```python
from build123d import *

# Parameters (mm, degrees)
F0_W     = 80
F0_H     = 55
F1_DEPTH = 10
F2_W     = 10
F2_H     = 10
F3_DEPTH = 5
F4_R     = 1


with BuildPart() as f1:
    # F0 (on Front) → F1 (new body)
    with BuildSketch(Plane.XZ):
        with Locations((-69.614079, 6.646032)):
            Rectangle(F0_W, F0_H)
    extrude(amount=F1_DEPTH)

    # F2 (on face) → F3 (cut)
    with BuildSketch(Plane.XZ.offset(10)):
        with Locations((-94.614079, 19.146032)):
            Rectangle(F2_W, F2_H)
        with Locations((-94.614079, -4.553968)):
            Rectangle(F2_W, F2_H)
        with Locations((-69.614079, 19.146032)):
            Rectangle(F2_W, F2_H)
        with Locations((-69.614079, -4.553968)):
            Rectangle(F2_W, F2_H)
        with Locations((-44.614079, 19.146032)):
            Rectangle(F2_W, F2_H)
        with Locations((-44.614079, -4.553968)):
            Rectangle(F2_W, F2_H)
    extrude(amount=-F3_DEPTH, mode=Mode.SUBTRACT)

    # F4
    f4_edges = [f1.edges().sort_by_distance(p)[0] for p in [
        (-69.614079, -10, 34.146032),
        (-29.614079, -10, 6.646032),
        (-109.614079, -10, 6.646032),
        (-69.614079, -10, -20.853968),
        (-89.614079, -10, -4.553968),
        (-94.614079, -10, 0.446032),
        (-99.614079, -10, -4.553968),
        (-94.614079, -10, -9.553968),
        (-64.614079, -10, -4.553968),
        (-69.614079, -10, 0.446032),
        (-74.614079, -10, -4.553968),
        (-69.614079, -10, -9.553968),
        (-39.614079, -10, -4.553968),
        (-44.614079, -10, 0.446032),
        (-49.614079, -10, -4.553968),
        (-44.614079, -10, -9.553968),
        (-89.614079, -10, 19.146032),
        (-94.614079, -10, 24.146032),
        (-99.614079, -10, 19.146032),
        (-94.614079, -10, 14.146032),
        (-64.614079, -10, 19.146032),
        (-69.614079, -10, 24.146032),
        (-74.614079, -10, 19.146032),
        (-69.614079, -10, 14.146032),
        (-39.614079, -10, 19.146032),
        (-44.614079, -10, 24.146032),
        (-49.614079, -10, 19.146032),
        (-44.614079, -10, 14.146032),
        (-69.614079, 0, 34.146032),
        (-109.614079, 0, 6.646032),
        (-69.614079, 0, -20.853968),
        (-29.614079, 0, 6.646032),
        (-29.614079, -5, 34.146032),
        (-29.614079, -5, -20.853968),
        (-109.614079, -5, 34.146032),
        (-109.614079, -5, -20.853968),
    ]]
    fillet(f4_edges, radius=F4_R)


solid = f1.part
```
Geometry: final body of the model. Coordinates: model frame, mm. Round coordinates to 2 decimals unless told otherwise and drop trailing zeros. Loops run counter-clockwise (first coordinate to the right, second up) from the corner with the lowest first, then second, coordinate; pieces in that order, holes last.
Item 1: Contact query for a flat-ended pin moving along its axis: P1, Ø5, axis at x = -71.5, z = -6.5, coming from the -Y side. Output: stop coordinate, or through.
Checked values:
P1: stops at y = -5
Item 2: Line query: L1, parallel to Z at x = -74, y = -6; L2, parallel to Y at x = -46, z = -0.5; L3, parallel to Y at x = -64, z = -9.5. Output: solid intervals per line, ascending.
Checked values:
L1: z = -20.85 to -9.55, 0.45 to 14.15, 24.15 to 34.15
L2: y = -5 to 0
L3: y = -9.92 to 0
Item 3: Mould query, pull axis Z, two halves, no side actions, for faces 1 (the flat face through (-29.614, -5, 6)), 2 (the flat face through (-70, -5, -20.854)), 3 (the flat face through (-45, -5, 19)). Classes: released by +Z, released by -Z, zero draft, split by the parting line, or undercut.
Checked values:
face 1: zero draft
face 2: released by -Z
face 3: undercut
Item 4: Section B-B, the plane z = 15. Output: boundary loops of the cut face in (x, y), plus the area to 3 significant figures.
Checked values:
outline: (-109.61, -9) arc R1 ccw to (-108.61, -10) - (-100.61, -10) arc R1 ccw to (-99.61, -9) - (-99.61, -5) - (-89.61, -5) - (-89.61, -9) arc R1 ccw to (-88.61, -10) - (-75.61, -10) arc R1 ccw to (-74.61, -9) - (-74.61, -5) - (-64.61, -5) - (-64.61, -9) arc R1 ccw to (-63.61, -10) - (-50.61, -10) arc R1 ccw to (-49.61, -9) - (-49.61, -5) - (-39.61, -5) - (-39.61, -9) arc R1 ccw to (-38.61, -10) - (-30.61, -10) arc R1 ccw to (-29.61, -9) - (-29.61, -1) arc R1 ccw to (-30.61, 0) - (-108.61, 0) arc R1 ccw to (-109.61, -1) - close
area: 648 mm2
Item 5: Section C-C, the plane x = -71.5. Output: boundary loops of the cut face in (y, z), plus the area to 3 significant figures.
Checked values:
outline: (-10, -19.85) arc R1 ccw to (-9, -20.85) - (-1, -20.85) arc R1 ccw to (0, -19.85) - (0, 33.15) arc R1 ccw to (-1, 34.15) - (-9, 34.15) arc R1 ccw to (-10, 33.15) - (-10, 25.15) arc R1 ccw to (-9, 24.15) - (-5, 24.15) - (-5, 14.15) - (-9, 14.15) arc R1 ccw to (-10, 13.15) - (-10, 1.45) arc R1 ccw to (-9, 0.45) - (-5, 0.45) - (-5, -9.55) - (-9, -9.55) arc R1 ccw to (-10, -10.55) - close
area: 448 mm2
Item 6: Section A-A, the plane y = -6.75. State how many separate pieces and enclosed holes the cut face has, plus the area to 3 significant figures.
Checked values:
separate pieces: 1
enclosed holes: 6
area: 3,800 mm2
